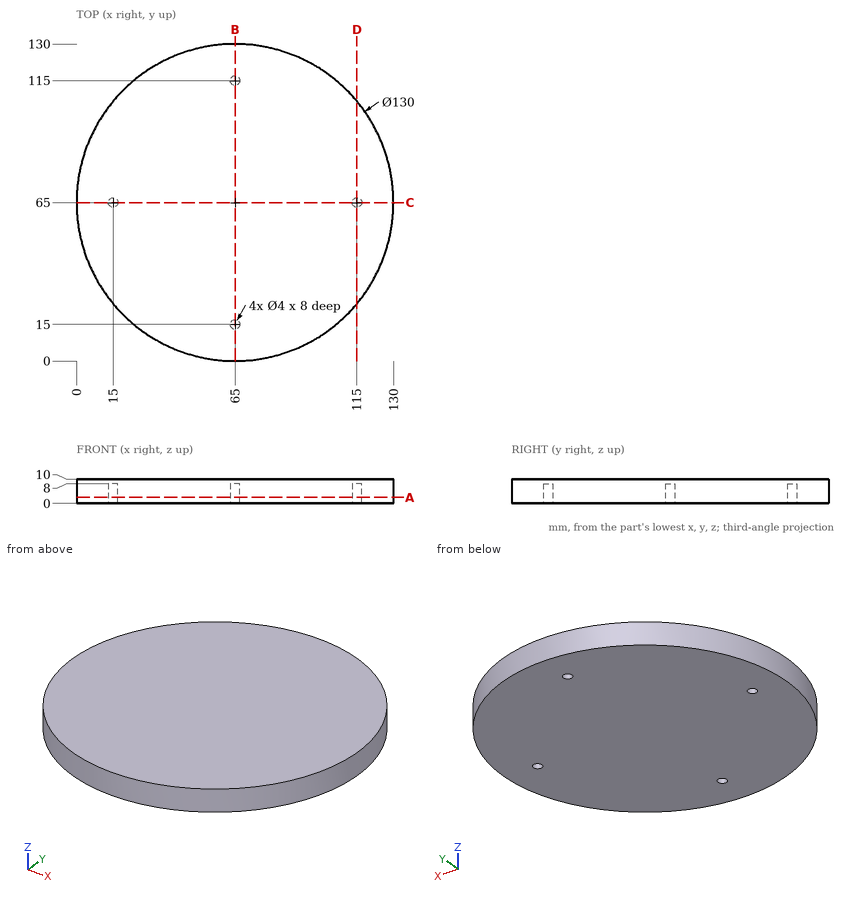
Drawing for the job (mm, zero at the part's lowest x, y, z). Round coordinates to 2 decimals unless told otherwise and drop trailing zeros. Write each loop counter-clockwise with the first axis right and the second up, starting at its lowest first coordinate (ties: lowest second). Pieces come first, ordered by that corner, then holes. Notation, with made-up numbers: (22, 63) - (49, 63) arc R16 ccw to (49, 88) - close; hole circle Ø2 at (-15, 61.25). An arc over 180 degrees is marked (long way). Use CSV: the item, a comma, the result in double quotes.
(1) Band-saw the part on B-B (x = 65). Write the cut outline in (y, z), plus the area to 3 significant figures.
Response:
outline,"(0, 0) - (13, 0) - (13, 8) - (17, 8) - (17, 0) - (113, 0) - (113, 8) - (117, 8) - (117, 0) - (130, 0) - (130, 10) - (0, 10) - close"
area,"1,240 mm²"
(2) Pin check, flat tips, straight feed: P1, Ø6.5, axis at x = 65, y = 15, coming from the -Z side; P2, Ø4, axis at y = 51.5, z = 4.5, coming from the -X side; P3, Ø1.2, axis at x = 64.5, y = 15.5, coming from the -Z side; P4, Ø2, axis at x = 61.5, z = 7, coming from the -Y side. Stop position of each tip, or through.
Response:
P1,"z = 0"
P2,"x = 1.03"
P3,"z = 8"
P4,"y = 0.05"
(3) Band-saw the part on A-A (z = 2.5). Write the cut outline in (x, y), plus the area to 3 significant figures.
Response:
outline,"circle Ø130 at (65, 65); hole circle Ø4 at (15, 65); hole circle Ø4 at (65, 15); hole circle Ø4 at (65, 115); hole circle Ø4 at (115, 65)"
area,"13,200 mm²"
(4) Band-saw the part on D-D (x = 115). Write the cut outline in (y, z), plus the area to 3 significant figures.
Response:
outline,"(23.47, 0) - (63, 0) - (63, 8) - (67, 8) - (67, 0) - (106.53, 0) - (106.53, 10) - (23.47, 10) - close"
area,"799 mm²"
(5) Wall check: line 1 (Y direction, x = 65, z = 5.5); line 2 (Y direction, x = 15, z = 2); line 3 (X direction, y = 15.5, z = 0.5). Give the ranges that are in metal, low to high.
Response:
line 1,"0 to 13, 17 to 113, 117 to 130"
line 2,"23.47 to 63, 67 to 106.53"
line 3,"22.87 to 63.06, 66.94 to 107.13"
